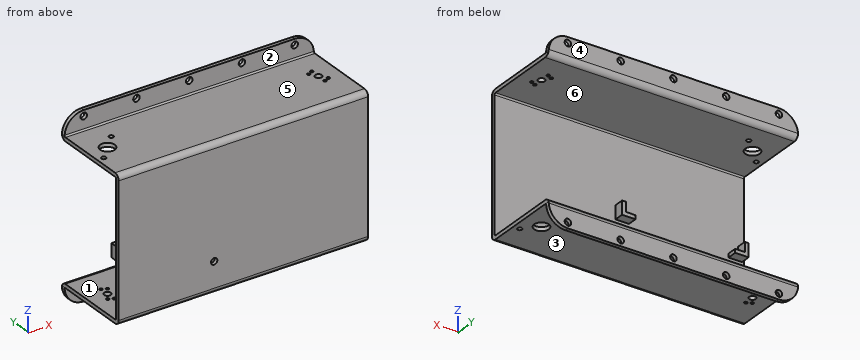
```python
from build123d import *

# Parameters (mm, degrees)
SKETCH_1_W                         = 130
SKETCH_1_H                         = 74.2
SM_BASE_FLANGE_1_DEPTH             = 2
SM_EDGE_FLANGE_1_STRIP_W           = 9.4732
SM_EDGE_FLANGE_1_STRIP_H           = 2
SM_EDGE_FLANGE_1_STRIP_CUT_DEPTH   = 130
SM_EDGE_FLANGE_1_STRIP_2_W         = 9.4732
SM_EDGE_FLANGE_1_STRIP_2_H         = 2
SM_EDGE_FLANGE_1_STRIP_CUT_2_DEPTH = 130
SM_EDGE_FLANGE_1_DEPTH             = 130
SM_EDGE_FLANGE_1_BEND_DEPTH        = 130
SM_EDGE_FLANGE_2_STRIP_W           = 9.4732
SM_EDGE_FLANGE_2_STRIP_H           = 2
SM_EDGE_FLANGE_2_STRIP_CUT_DEPTH   = 130
SM_EDGE_FLANGE_2_STRIP_2_W         = 9.4732
SM_EDGE_FLANGE_2_STRIP_2_H         = 2
SM_EDGE_FLANGE_2_STRIP_CUT_2_DEPTH = 130
SM_EDGE_FLANGE_2_DEPTH             = 130
SM_EDGE_FLANGE_2_BEND_DEPTH        = 130
HOLE_WIZARD_M1_4_1_D               = 1.6
HOLE_WIZARD_M1_4_1_DEPTH           = 2
HOLE_WIZARD_M1_4_2_D               = 1.6
HOLE_WIZARD_M1_4_2_DEPTH           = 2
HOLE_WIZARD_3_5_3_5_1_D            = 3.5
HOLE_WIZARD_3_5_3_5_1_DEPTH        = 2
HOLE_WIZARD_3_5_3_5_2_D            = 3.5
HOLE_WIZARD_3_5_3_5_2_DEPTH        = 2
HOLE_WIZARD_7_7_7_7_1_D            = 7.7
HOLE_WIZARD_7_7_7_7_1_DEPTH        = 2
HOLE_WIZARD_7_7_7_7_2_D            = 7.7
HOLE_WIZARD_7_7_7_7_2_DEPTH        = 2
HOLE_WIZARD_M3_2_D                 = 3.4
EXTRUDE_1_DEPTH                    = 5
HOLE_WIZARD_M2_4_D                 = 2.4
HOLE_WIZARD_M2_4_DEPTH             = 2
HOLE_WIZARD_M2_5_D                 = 2.4
HOLE_WIZARD_M2_5_DEPTH             = 2
HOLE_WIZARD_M3_3_D                 = 3.4
HOLE_WIZARD_M3_3_DEPTH             = 1.978536948
HOLE_WIZARD_M3_3_TIP               = 1.021463052
FILLET_1_R                         = 10


# Sheet-metal steps are written as plain solids
with BuildPart() as part:
    # Sketch 1 → 基体-法兰1 (new body)
    with BuildSketch(Plane(origin=(0, 0, 0), x_dir=(1, 0, 0), z_dir=(0, 1, 0))):
        Rectangle(SKETCH_1_W, SKETCH_1_H)
    extrude(amount=-SM_BASE_FLANGE_1_DEPTH)

    # 边线-法兰1 strip (across the edge) → 边线-法兰1 strip cut (cut)
    with BuildSketch(Plane(origin=(-65, 0, 37.1), x_dir=(0, 0, -1), z_dir=(1, 0, 0))):
        with Locations((-2, -1)):
            Rectangle(SM_EDGE_FLANGE_1_STRIP_W, SM_EDGE_FLANGE_1_STRIP_H)
    extrude(amount=SM_EDGE_FLANGE_1_STRIP_CUT_DEPTH, mode=Mode.SUBTRACT)

    # 边线-法兰1 strip 2 (across the edge) → 边线-法兰1 strip cut 2 (cut)
    with BuildSketch(Plane(origin=(65, 0, -37.1), x_dir=(0, 0, 1), z_dir=(-1, 0, 0))):
        with Locations((-2, -1)):
            Rectangle(SM_EDGE_FLANGE_1_STRIP_2_W, SM_EDGE_FLANGE_1_STRIP_2_H)
    extrude(amount=SM_EDGE_FLANGE_1_STRIP_CUT_2_DEPTH, mode=Mode.SUBTRACT)

    # 边线-法兰1 section (across the edge) → 边线-法兰1 (add)
    with BuildSketch(Plane(origin=(-65, 0, 37.1), x_dir=(0, 0, -1), z_dir=(1, 0, 0))):
        with BuildLine():
            Line((0, 0.7366), (0, 41))
            Line((0, 41), (2, 41))
            Line((2, 41), (2, 0.7366))
            ThreePointArc((2, 0.7366), (2.215745145, 0.215745145), (2.7366, 0))
            Line((2.7366, 0), (2.7366, -2))
            ThreePointArc((2.7366, -2), (0.801531583, -1.198468417), (0, 0.7366))
        make_face()
    extrude(amount=SM_EDGE_FLANGE_1_DEPTH)

    # 边线-法兰1 section 2 (across the edge) → 边线-法兰1 bend (add)
    with BuildSketch(Plane(origin=(65, 0, -37.1), x_dir=(0, 0, 1), z_dir=(-1, 0, 0))):
        with BuildLine():
            Line((0, 0.7366), (0, 41))
            Line((0, 41), (2, 41))
            Line((2, 41), (2, 0.7366))
            ThreePointArc((2, 0.7366), (2.215745145, 0.215745145), (2.7366, 0))
            Line((2.7366, 0), (2.7366, -2))
            ThreePointArc((2.7366, -2), (0.801531583, -1.198468417), (0, 0.7366))
        make_face()
    extrude(amount=SM_EDGE_FLANGE_1_BEND_DEPTH)

    # 边线-法兰2 strip (across the edge) → 边线-法兰2 strip cut (cut)
    with BuildSketch(Plane(origin=(65, 41, 37.1), x_dir=(0, -1, 0), z_dir=(-1, 0, 0))):
        with Locations((-2, -1)):
            Rectangle(SM_EDGE_FLANGE_2_STRIP_W, SM_EDGE_FLANGE_2_STRIP_H)
    extrude(amount=SM_EDGE_FLANGE_2_STRIP_CUT_DEPTH, mode=Mode.SUBTRACT)

    # 边线-法兰2 strip 2 (across the edge) → 边线-法兰2 strip cut 2 (cut)
    with BuildSketch(Plane(origin=(-65, 41, -37.1), x_dir=(0, -1, 0), z_dir=(1, 0, 0))):
        with Locations((-2, -1)):
            Rectangle(SM_EDGE_FLANGE_2_STRIP_2_W, SM_EDGE_FLANGE_2_STRIP_2_H)
    extrude(amount=SM_EDGE_FLANGE_2_STRIP_CUT_2_DEPTH, mode=Mode.SUBTRACT)

    # 边线-法兰2 section (across the edge) → 边线-法兰2 (add)
    with BuildSketch(Plane(origin=(65, 41, 37.1), x_dir=(0, -1, 0), z_dir=(-1, 0, 0))):
        with BuildLine():
            Line((0, 0.7366), (0, 10))
            Line((0, 10), (2, 10))
            Line((2, 10), (2, 0.7366))
            ThreePointArc((2, 0.7366), (2.215745145, 0.215745145), (2.7366, 0))
            Line((2.7366, 0), (2.7366, -2))
            ThreePointArc((2.7366, -2), (0.801531583, -1.198468417), (0, 0.7366))
        make_face()
    extrude(amount=SM_EDGE_FLANGE_2_DEPTH)

    # 边线-法兰2 section 2 (across the edge) → 边线-法兰2 bend (add)
    with BuildSketch(Plane(origin=(-65, 41, -37.1), x_dir=(0, -1, 0), z_dir=(1, 0, 0))):
        with BuildLine():
            Line((0, 0.7366), (0, 10))
            Line((0, 10), (2, 10))
            Line((2, 10), (2, 0.7366))
            ThreePointArc((2, 0.7366), (2.215745145, 0.215745145), (2.7366, 0))
            Line((2.7366, 0), (2.7366, -2))
            ThreePointArc((2.7366, -2), (0.801531583, -1.198468417), (0, 0.7366))
        make_face()
    extrude(amount=SM_EDGE_FLANGE_2_BEND_DEPTH)

    # M1.4 间隙孔1
    with Locations(Plane(origin=(0, 0, -37.1), x_dir=(-1, 0, 0), z_dir=(0, 0, -1))):
        with Locations((52.5, 24.75), (55, 26), (57.5, 17.25), (55, 16)):
            Hole(HOLE_WIZARD_M1_4_1_D / 2, depth=HOLE_WIZARD_M1_4_1_DEPTH)

    # M1.4 间隙孔2
    with Locations(Plane.XY.offset(37.1)):
        with Locations((52.5, 24.75), (55, 26), (57.5, 17.25), (55, 16)):
            Hole(HOLE_WIZARD_M1_4_2_D / 2, depth=HOLE_WIZARD_M1_4_2_DEPTH)

    # Ø3.5 (3.5) 直径孔1
    with Locations(Plane(origin=(0, 0, -37.1), x_dir=(-1, 0, 0), z_dir=(0, 0, -1))):
        with Locations((55, 21)):
            Hole(HOLE_WIZARD_3_5_3_5_1_D / 2, depth=HOLE_WIZARD_3_5_3_5_1_DEPTH)

    # Ø3.5 (3.5) 直径孔2
    with Locations(Plane.XY.offset(37.1)):
        with Locations((55, 21)):
            Hole(HOLE_WIZARD_3_5_3_5_2_D / 2, depth=HOLE_WIZARD_3_5_3_5_2_DEPTH)

    # Ø7.7 (7.7) 直径孔1
    with Locations(Plane(origin=(0, 0, -37.1), x_dir=(-1, 0, 0), z_dir=(0, 0, -1))):
        with Locations((-55, 21)):
            Hole(HOLE_WIZARD_7_7_7_7_1_D / 2, depth=HOLE_WIZARD_7_7_7_7_1_DEPTH)

    # Ø7.7 (7.7) 直径孔2
    with Locations(Plane.XY.offset(37.1)):
        with Locations((-55, 21)):
            Hole(HOLE_WIZARD_7_7_7_7_2_D / 2, depth=HOLE_WIZARD_7_7_7_7_2_DEPTH)

    # M3 间隙孔2 (through all)
    with Locations(Plane(origin=(0, 41, 0), x_dir=(1, 0, 0), z_dir=(0, 1, 0))):
        with Locations((-55, 44.1), (-27.5, 44.1), (27.5, 44.1), (55, 44.1), (55, -44.1), (27.5, -44.1), (0, -44.1), (-27.5, -44.1), (-55, -44.1), (0, 44.1)):
            Hole(HOLE_WIZARD_M3_2_D / 2)

    # 草图46 → 凸台-拉伸1 (add)
    with BuildSketch(Plane(origin=(0, 0, 0), x_dir=(1, 0, 0), z_dir=(0, 1, 0))):
        Polygon((1.974724409, 6.87), (-5.025275591, 6.87), (-5.025275591, 4.87), (-0.025275591, 4.87), (-0.025275591, -0.13), (1.974724409, -0.13), align=None)
        Polygon((-64, 6.87), (-64, -0.13), (-62, -0.13), (-62, 4.87), (-57, 4.87), (-57, 6.87), align=None)
    extrude(amount=EXTRUDE_1_DEPTH)

    # M2 间隙孔4
    with Locations(Plane(origin=(0, 0, -37.1), x_dir=(-1, 0, 0), z_dir=(0, 0, -1))):
        with Locations((-48.366748111, 27.800733003), (-61.633251889, 14.199266997)):
            Hole(HOLE_WIZARD_M2_4_D / 2, depth=HOLE_WIZARD_M2_4_DEPTH)

    # M2 间隙孔5
    with Locations(Plane(origin=(0, 0, 35.1), x_dir=(-1, 0, 0), z_dir=(0, 0, -1))):
        with Locations((48.366748111, 27.800733003), (61.633251889, 14.199266997)):
            Hole(HOLE_WIZARD_M2_5_D / 2, depth=HOLE_WIZARD_M2_5_DEPTH)

    # M3 间隙孔3
    with Locations(Plane(origin=(0, 0, 0), x_dir=(1, 0, 0), z_dir=(0, 1, 0))):
        with Locations((-15.23, 21.09)):
            Hole(HOLE_WIZARD_M3_3_D / 2, depth=HOLE_WIZARD_M3_3_DEPTH)
            with Locations((0, 0, -(HOLE_WIZARD_M3_3_DEPTH + HOLE_WIZARD_M3_3_TIP / 2))):  # 118° drill point
                Cone(0, HOLE_WIZARD_M3_3_D / 2, HOLE_WIZARD_M3_3_TIP, mode=Mode.SUBTRACT)

    # 圆角1
    fillet_1_edges = [part.edges().sort_by_distance(p)[0] for p in [
        (65, 40, -47.1),
        (65, 40, 47.1),
        (-65, 40, 47.1),
        (-65, 40, -47.1),
    ]]
    fillet(fillet_1_edges, radius=FILLET_1_R - 0.0001)  # a hair under: the kernel refuses the full size


solid = part.part
```
Build history of the part. All positions in model axes, mm. Face numbers are marked on the shaded views. A direction names the side the tool comes from. Round coordinates to 2 decimals unless told otherwise and drop trailing zeros. Loops run counter-clockwise (first coordinate to the right, second up) from the corner with the lowest first, then second, coordinate; pieces in that order, holes last.
Item 1: Pin check, flat tips, straight feed: P1, Ø2, axis at x = -50.5, z = -33.5, coming from the +Y side; P2, Ø4, axis at x = -55, y = 21, coming from the -Z side; P3, Ø8, axis at x = 5, y = 21, coming from the +Z side; P4, Ø5.5, axis at x = -55, z = -44.1, coming from the +Y side. Stop position of each tip, or through.
Item 2: Drill centre lines: line 1 along Z through (x, y) = (20, 4.5); line 2 along Y through (x, z) = (55, 36.4); line 3 along X through (y, z) = (39.5, -44.1). Where is each one in solid material? Low to high.
Item 3: Saw through at A-A (y = 10.5). List the corners of the cut face in (x, z), then the cut area to 3 significant figures.
Item 4: Saw through at D-D (z = -3). List the corners of the cut face in (x, y).
Item 5: Two-plate mould, pull along Z, no slides. Class the marked faces 1, 2 and 3: released by +Z, released by -Z, zero draft, split by the parting line, or undercut.
Item 6: Which spindle directions (+Z, -Z, +X, -X, +Y, -Y) get a long thin tool onto all of the face, cutting with end or side? Do the marked faces 4, 5 and 6. Say none if no direction does.
Item 7: Saw through at C-C (x = -21). List the corners of the cut face in (y, z).
Item 8: Saw through at B-B (z = 44.1). List the corners of the cut face in (x, y).
Worked answers:
1. P1: stops at y = 0.01
1. P2: stops at z = -37.1
1. P3: stops at z = 37.1
1. P4: stops at y = 41
2. line 1: z = -37.1 to -35.1, 35.1 to 37.1
2. line 2: y = -1.09 to 15.2, 16.8 to 19.25, 22.75 to 25.2, 26.8 to 40.59
2. line 3: x = -62.14 to -56.7, -53.3 to -29.2, -25.8 to -1.7, 1.7 to 25.8, 29.2 to 53.3, 56.7 to 62.14
3. outline: (-65, -37.1) - (65, -37.1) - (65, -35.1) - (-65, -35.1) - close; (-65, 35.1) - (65, 35.1) - (65, 37.1) - (-65, 37.1) - close
3. area: 520 mm2
4. outline: (-65, -2) - (65, -2) - (65, 0) - (1.97, 0) - (1.97, 5) - (-0.03, 5) - (-0.03, 0) - (-62, 0) - (-62, 5) - (-64, 5) - (-64, 0) - (-65, 0) - close
5. face 1: undercut
5. face 2: zero draft
5. face 3: released by -Z
6. face 4: +Z, -Z, +X, -X, +Y
6. face 5: +Z, +X, -X, -Y
6. face 6: +X, -X, +Y
7. outline: (-2, -34.36) arc R2.74 ccw to (0.74, -37.1) - (38.26, -37.1) arc R0.74 cw to (39, -37.84) - (39, -47.1) - (41, -47.1) - (41, -37.84) arc R2.74 ccw to (38.26, -35.1) - (0.74, -35.1) arc R0.74 cw to (0, -34.36) - (0, 34.36) arc R0.74 cw to (0.74, 35.1) - (38.26, 35.1) arc R2.74 ccw to (41, 37.84) - (41, 47.1) - (39, 47.1) - (39, 37.84) arc R0.74 cw to (38.26, 37.1) - (0.74, 37.1) arc R2.74 ccw to (-2, 34.36) - close
8. outline: (-62.14, 39) - (-56.7, 39) - (-56.7, 41) - (-62.14, 41) - close; (-53.3, 39) - (-29.2, 39) - (-29.2, 41) - (-53.3, 41) - close; (-25.8, 39) - (-1.7, 39) - (-1.7, 41) - (-25.8, 41) - close; (1.7, 39) - (25.8, 39) - (25.8, 41) - (1.7, 41) - close; (29.2, 39) - (53.3, 39) - (53.3, 41) - (29.2, 41) - close; (56.7, 39) - (62.14, 39) - (62.14, 41) - (56.7, 41) - close
